Read the model definition and answer for the solid it produces. Units are mm, in the model's axes. Coordinates: 2 decimals unless noted, no trailing zeros. Loops run counter-clockwise (first coordinate to the right, second up) from the corner with the lowest first, then second, coordinate; pieces in that order, holes last.
from build123d import *

# Parameters (mm, degrees)
SKETCH_1_R      = 0.75
EXTRUDE_2_DEPTH = 1


with BuildPart() as part:
    # 草图1 → 凸台-拉伸2 (new body)
    with BuildSketch(Plane(origin=(0, 0, 0), x_dir=(1, 0, 0), z_dir=(0, 1, 0))):
        with BuildLine():
            Line((23.799708029, 17.537518248), (-53.200291971, 17.537518248))
            ThreePointArc((-53.200291971, 17.537518248), (-54.473084177, 17.010310454), (-55.000291971, 15.737518248))
            Line((-55.000291971, 15.737518248), (-55.000291971, -21.162481752))
            ThreePointArc((-55.000291971, -21.162481752), (-54.473084177, -22.435273958), (-53.200291971, -22.962481752))
            Line((-53.200291971, -22.962481752), (55.999708029, -22.962481752))
            ThreePointArc((55.999708029, -22.962481752), (57.272500235, -22.435273958), (57.799708029, -21.162481752))
            Line((57.799708029, -21.162481752), (57.799708029, 15.737518248))
            ThreePointArc((57.799708029, 15.737518248), (57.272500235, 17.010310454), (55.999708029, 17.537518248))
            Line((55.999708029, 17.537518248), (55.799708029, 17.537518248))
            Line((55.799708029, 17.537518248), (55.799708029, 7.537518248))
            Line((55.799708029, 7.537518248), (41.799708029, 7.537518248))
            Line((41.799708029, 7.537518248), (41.799708029, 17.537518248))
            Line((41.799708029, 17.537518248), (37.799708029, 17.537518248))
            Line((37.799708029, 17.537518248), (37.799708029, 7.537518248))
            Line((37.799708029, 7.537518248), (23.799708029, 7.537518248))
            Line((23.799708029, 7.537518248), (23.799708029, 17.537518248))
        make_face()
        with Locations(Location((-53.200291971, -21.162481752, 0), (0, 0, 270))):
            Circle(SKETCH_1_R, mode=Mode.SUBTRACT)
        with Locations(Location((20.549708029, -2.712481752, 0), (0, 0, 270))):
            Circle(SKETCH_1_R, mode=Mode.SUBTRACT)
        with Locations(Location((-53.200291971, 15.737518248, 0), (0, 0, 270))):
            Circle(SKETCH_1_R, mode=Mode.SUBTRACT)
    extrude(amount=EXTRUDE_2_DEPTH)


solid = part.part
Q1. A cutting plane is placed at C-C (x = 30). Give the vertices of the cut face in (y, z), then the cut area to 3 significant figures.
Findings below:
outline: (0, -7.54) - (1, -7.54) - (1, 22.96) - (0, 22.96) - close
area: 30.5 mm2
Q2. A cutting plane is placed at A-A (z = -13). Give the vertices of the cut face in (x, y).
Findings below:
outline: (-55, 0) - (23.8, 0) - (23.8, 1) - (-55, 1) - close; (37.8, 0) - (41.8, 0) - (41.8, 1) - (37.8, 1) - close; (55.8, 0) - (57.8, 0) - (57.8, 1) - (55.8, 1) - close
Q3. A flat-ended cylindrical pin translates along its axis: pin 1 Ø1.4 at (x, z) = (20.55, 2.71) entering from +Y. Find the tip coordinate at first contact, or state that the pin passes through.
Findings below:
pin 1: passes through
Q4. A cutting plane is placed at B-B (y = 0.3). Give the vertices of the cut face in (x, z).
Findings below:
outline: (-55, -15.74) arc R1.8 ccw to (-53.2, -17.54) - (23.8, -17.54) - (23.8, -7.54) - (37.8, -7.54) - (37.8, -17.54) - (41.8, -17.54) - (41.8, -7.54) - (55.8, -7.54) - (55.8, -17.54) - (56, -17.54) arc R1.8 ccw to (57.8, -15.74) - (57.8, 21.16) arc R1.8 ccw to (56, 22.96) - (-53.2, 22.96) arc R1.8 ccw to (-55, 21.16) - close; hole circle Ø1.5 at (-53.2, -15.74); hole circle Ø1.5 at (-53.2, 21.16); hole circle Ø1.5 at (20.55, 2.71)
Q5. Straight lines are drawn through the part: probe 1 along Z at (x, y) = (51.5, 0.95); probe 2 along X at (y, z) = (0.3, 2.5); probe 3 along X at (y, z) = (0.85, 20.5). For each, find the intervals that lie inside material, in ascending order.
Findings below:
probe 1: z = -7.54 to 22.96
probe 2: x = -55 to 19.83, 21.27 to 57.8
probe 3: x = -55 to -53.55, -52.85 to 57.8
